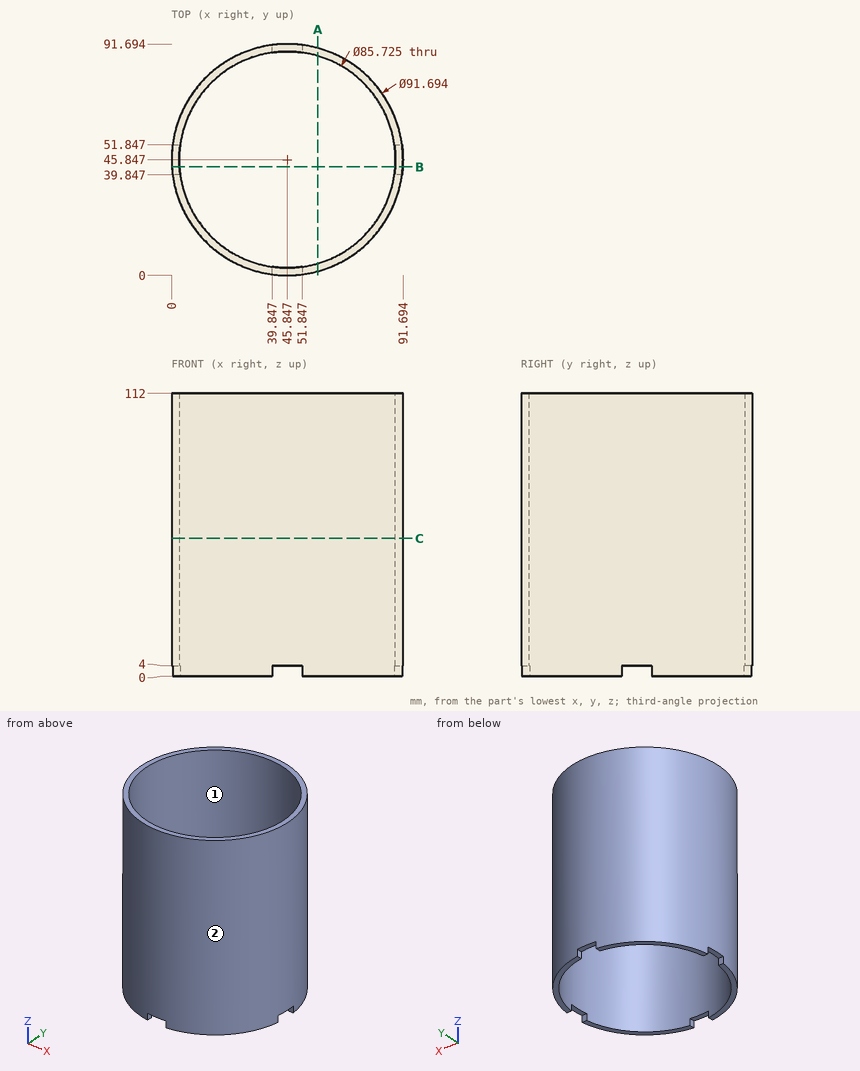
The figure shows three views and two pictorial views of one solid part (mm, origin at its lowest corner). Answer the questions. Give positions to 0.01 mm unless a question says otherwise; leave off trailing zeros. Order: outer loops, then holes, each group sorted by start corner. A loop starts at its lowest first (then second) coordinate and runs counter-clockwise, first axis right, second up. Notation, with made-up numbers: (-12, 45.5) - (2, 45.5) arc R15 ccw to (2, 72.5) - close; hole circle Ø1 at (38.5, 52.25). An arc over 180 degrees is marked (long way). Answer as CSV lines item,"result".
Q1. Each of these flat-tipped pins is pushed along its axis until it touches: pin 1 Ø2 at (y, z) = (43.5, 57.5) entering from +X; pin 2 Ø2.5 at (y, z) = (89.5, 1.5) entering from -X; pin 3 Ø1 at (x, y) = (45, 90) entering from -Z. Where does it stop, or does it pass through?
Answer key:
pin 1,"stops at x = 91.67"
pin 2,"stops at x = 28.41"
pin 3,"stops at z = 4"
Q2. Straight lines are drawn through the part: L1, parallel to Y at x = 40, z = 81; L2, parallel to X at y = 45.5, z = 103; L3, parallel to X at y = 76, z = 101. For each, find the intervals that lie inside material, in ascending order.
Answer key:
L1,"y = 0.37 to 3.39, 88.31 to 91.32"
L2,"x = 0 to 2.99, 88.71 to 91.69"
L3,"x = 11.31 to 15.38, 76.31 to 80.38"
Q3. A cutting plane is placed at B-B, the plane y = 43. Determine the outline of the cut face in (x, z), and give its area (3 significant figures).
Answer key:
outline,"(0.09, 4) - (3.08, 4) - (3.08, 112) - (0.09, 112) - close; (88.61, 4) - (91.61, 4) - (91.61, 112) - (88.61, 112) - close"
area,"646 mm^2"
Q4. A cutting plane is placed at C-C, the plane z = 54.5. Determine the outline of the cut face in (x, y) (1 decimal).
Answer key:
outline,"circle Ø91.7 at (45.8, 45.8); hole circle Ø85.7 at (45.8, 45.8)"
Q5. A cutting plane is placed at A-A, the plane x = 58. Determine the outline of the cut face in (y, z).
Answer key:
outline,"(1.64, 0) - (4.74, 0) - (4.74, 112) - (1.64, 112) - close; (86.95, 0) - (90.05, 0) - (90.05, 112) - (86.95, 112) - close"
Q6. Determine the mould class of the marked faces 1 and 2 for opening direction Y: pulls with the +Y half, pulls with the -Y half, needs draft (parallel to the pull), parting line crosses it, or undercut.
Answer key:
face 1,"undercut"
face 2,"parting line crosses it"
